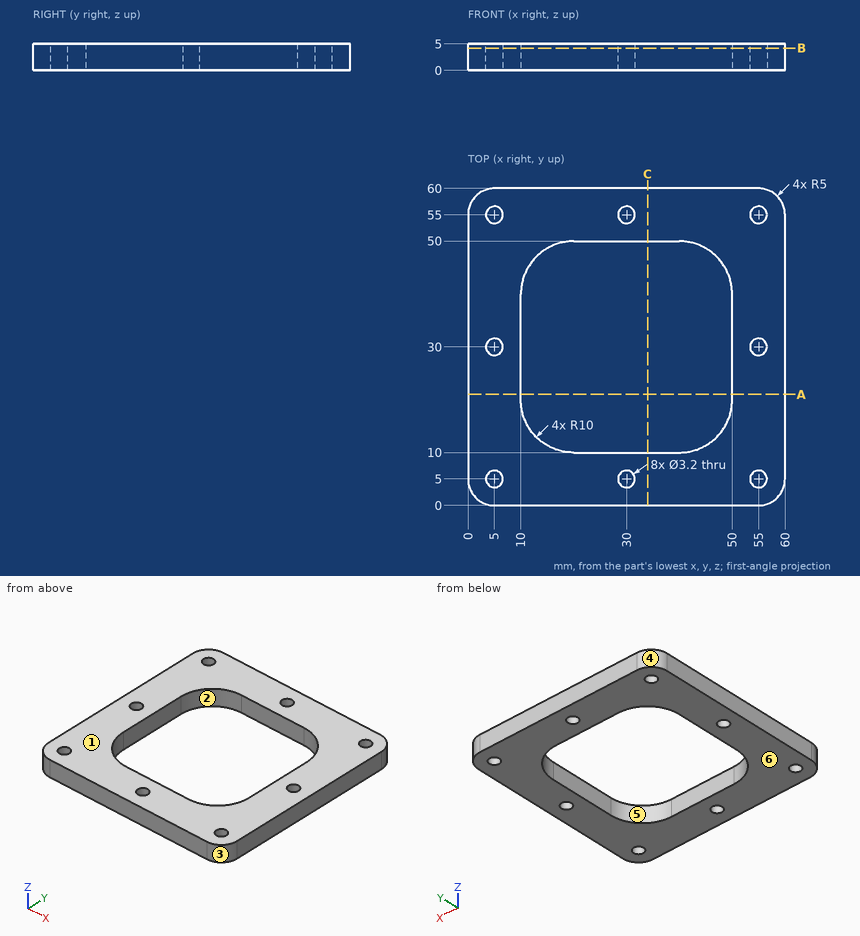
The drawing under review shows one solid part. Ordinate dimensions are in mm from its lowest x, y, z. A direction names the side the tool comes from. Round coordinates to 2 decimals unless told otherwise and drop trailing zeros. Write each loop counter-clockwise with the first axis right and the second up, starting at its lowest first coordinate (ties: lowest second). Pieces come first, ordered by that corner, then holes. Notation, with made-up numbers: (84, 85) - (105, 85) arc R23 cw to (105, 122) - close; hole circle Ø1 at (28.5, -21). An arc over 180 degrees is marked (long way). Write each question's results on one line, items separated by ' | '.
Item 1: Take a section at A-A on y = 21. State the section outline as (x, z) points.
Calculated:
outline: (0, 0) - (10, 0) - (10, 5) - (0, 5) - close; (50, 0) - (60, 0) - (60, 5) - (50, 5) - close
Item 2: Take a section at B-B on z = 4.2. Count the separate pieces of the cut face and the enclosed holes in it, then the cut area to 3 significant figures.
Calculated:
separate pieces: 1 | enclosed holes: 9 | area: 2,000 mm^2
Item 3: For the marked faces 5 and 6, list the 3-axis set-ups (+Z, -Z, +X, -X, +Y, -Y) from which the entire face can be reached by the end or side of a thin tool; tool diameter is ignored.
Calculated:
face 5: +Z, -Z | face 6: -Z, +X, -X, +Y, -Y
Item 4: Draft analysis for pull direction X (two halves, no side actions). For the marked faces 1, 2, 3 and 4, state which applies: pulls with the +X half, pulls with the -X half, needs draft (parallel to the pull), parting line crosses it, or undercut.
Calculated:
face 1: needs draft | face 2: undercut | face 3: pulls with the +X half | face 4: pulls with the -X half
Item 5: To check wall thickness, follow line 1 along Y through (x, z) = (55, 3.1); line 2 along Y through (x, z) = (37.5, 0.65). State the ranges of each line that lie inside material, in increasing order. Write a range as from..to.
Calculated:
line 1: y = 0..3.4, 6.6..28.4, 31.6..53.4, 56.6..60 | line 2: y = 0..10, 50..60
